Autodesk Inventor part; units mm, degrees
ref_plane "YZ Plane" through (0, 0, 0) normal (1, 0, 0) x (0, 1, 0)
ref_plane "XZ Plane" through (0, 0, 0) normal (0, 1, 0) x (-1, 0, 0)
ref_plane "XY Plane" through (0, 0, 0) normal (0, 0, 1) x (1, 0, 0)
sketch "Sketch1" plane through (0, 0, 0) normal (0, 0, 1) x (1, 0, 0)
  arc A0 (-1.508, 2.794) -> (-1.508, -2.794) centre (0, 0) ccw
  line L0 (-3.175, 0) -> (0, 0) construction
  line L1 (0, 0) -> (3.175, 0) construction
  line L2 (-1.508, 2.794) -> (1.508, 2.794)
  line L3 (-1.508, -2.794) -> (1.508, -2.794)
  arc A1 (1.508, 2.794) -> (-1.508, 2.794) centre (0, 0) ccw construction
  arc A2 (1.508, -2.794) -> (1.508, 2.794) centre (0, 0) ccw
  arc A3 (-1.508, -2.794) -> (1.508, -2.794) centre (0, 0) ccw construction
  circle A4 centre (0, 0) radius 3.429 construction
  circle A5 centre (0, 0) radius 4.064
  circle A6 centre (0, 0) radius 11.1125
  dimension "d1" = 2.794
  dimension "d2" = 3.175
  dimension "d3" = 6.858
  dimension "d5" = 0.635
  dimension "d6" = 22.225
extrude "Extrusion1" add sketch "Sketch1" along normal blind 3.048 contours A5 | A6
sketch "Sketch2" plane through (0, 0, 3.048) normal (0, 0, 1) x (1, 0, 0)
  circle A0 centre (0, 0) radius 11.1125
  arc A1 (-1.508, 2.794) -> (-1.508, -2.794) centre (0, 0) ccw
extrude "Extrusion2" add sketch "Sketch2" along normal blind 3.175
hole "Hole1" at (0, 0, 3.048) direction (0, 0, 1) diameter 3.302 depth 25.4 tip angle 118
sketch "Sketch3" plane through (0, 0, 6.223) normal (0, 0, 1) x (1, 0, 0)
  circle A0 centre (0, 0) radius 11.1125
  circle A1 centre (0, 0) radius 3.429
  circle A2 centre (0, 0) radius 4.064
  dimension "d18" = 6.858
  dimension "d19" = 0.635
extrude "Extrusion3" add sketch "Sketch3" along normal blind 6.1341 contours A0
chamfer "Chamfer1" distance 6.35 distance2 12.3571 1 edges at (-11.1125, 0, 0) measured on face at (0.4465, -5.5398, 0)
sketch "Sketch6" plane through (0, 0, 12.3571) normal (0, 0, 1) x (1, 0, 0)
  circle A0 centre (0, 0) radius 11.1125
  circle A1 centre (0, 0) radius 6.35
  circle A2 centre (0, 0) radius 8.7312
  dimension "d38" = 12.7
  dimension "d52" = 2.3813
  dimension "d53" = 2.3813
extrude "Extrusion5" add sketch "Sketch6" along normal blind 4.9784 contours A2
sketch "Sketch7" plane through (0, 0, 0) normal (1, 0, 0) x (0, 1, 0)
  line L0 (-6.35, 17.3355) -> (6.35, 17.3355)
  line L1 (6.35, 12.3571) -> (-6.35, 12.3571)
  line L2 (0, 0) -> (0, 12.3571) construction
  line L3 (0, 12.3571) -> (0, 17.3355) construction
  point P0 (0, 14.8463)
hole "Hole3" at (0, 0, 14.8463) direction (-1, 0, 0) diameter 2.159 end through all
sketch "Sketch8" plane through (0, 0, 12.3571) normal (0, 0, 1) x (1, 0, 0)
  circle A0 centre (0, 0) radius 11.1125
  circle A1 centre (0, 0) radius 8.7312
  line L0 (-10.3187, 4.1244) -> (-10.3188, -4.1244)
  line L1 (-11.1125, 0) -> (0, 0)
  dimension "d49" = 0.7937
extrude "Extrusion6" cut sketch "Sketch8" against normal through all contours L0 L1 A0 | A0 L1 L0
mirror "Mirror2" about plane through (0, 0, 0) normal (1, 0, 0) of "Hole3", "Extrusion6"
ref_plane "Work Plane2" through (0, 0, 4.953) normal (0, 0, -1) x (-1, 0, 0)
sketch "Sketch9" plane through (0, 0, 4.953) normal (0, 0, -1) x (-1, 0, 0)
  point P0 (0, 0)
equation "\"d52\" = d53"
properties part number "Pneumatic Connector -Actuator Side"
Verification items for the finished model (mm, model axes). A direction names the side the tool comes from. Give positions to 0.01 mm unless a question says otherwise; leave off trailing zeros. Loops run counter-clockwise (first coordinate to the right, second up) from the corner with the lowest first, then second, coordinate; pieces in that order, holes last.
1) Depth check by flat-ended pin: pin 1 Ø1.5 at (y, z) = (-7.5, 8) entering from -X; pin 2 Ø1.9 at (y, z) = (0, 14.85) entering from +X; pin 3 Ø6.5 at (x, y) = (-0.5, -1.5) entering from +Z; pin 4 Ø2.5 at (y, z) = (0, 14.85) entering from -X. Enter the tip coordinate at first touch or a pass-through.
2) Sectioned sample at D-D, the plane z = 4.5. Enter the section's corners in (x, y).
3) Sectioned sample at A-A, the plane y = 0. Count the separate pieces of the cut face and the enclosed holes in it, then the cut area to 3 significant figures.
4) Sectioned sample at C-C, the plane z = 14.5. Enter the section's corners in (x, y), then the cut area to 3 significant figures.
5) Draft check along Y on faces 1 (the flat face through (-6, -3, 17.336)), 2 (the cylindrical face through (7.512, -0.413, 13.849)), 3 (the cylindrical face through (0.632, 1.525, 4.658)), 4 (the conical face through (6.07, -2.52, 3.52)). Enter one of: pulls with the +Y half, pulls with the -Y half, needs draft (parallel to the pull), parting line crosses it, or undercut.
6) Set-up check for faces 5 (the cylindrical face through (-3.175, -0.048, 1.503)), 6 (the flat face through (-7, 6, 12.357)), 7 (the flat face through (0, -3, 0)): record each of +Z, -Z, +X, -X, +Y, -Y from which the full face is reachable in a straight line by a thin tool's end or side.
7) Thickness scan on line 1 along Y through (x, z) = (0, 14.95); line 2 along X through (y, z) = (1.25, 8); line 3 along Y through (x, z) = (-2, 3). Record the ranges inside material, lowest first.
Answers:
1. pin 1: stops at x = -5.94
1. pin 2: passes through
1. pin 3: stops at z = 12.36
1. pin 4: stops at x = -8.73
2. outline: circle Ø14.15 at (0, 0); hole circle Ø3.3 at (0, 0)
3. separate pieces: 4
3. enclosed holes: 0
3. area: 129 mm2
4. outline: (-8.67, -1.02) arc R8.73 ccw to (8.67, -1.02) - (6.27, -1.02) arc R6.35 cw to (-6.27, -1.02) - close; (-8.67, 1.02) - (-6.27, 1.02) arc R6.35 cw to (6.27, 1.02) - (8.67, 1.02) arc R8.73 ccw to start
4. area: 103 mm2
5. face 1: needs draft
5. face 2: undercut
5. face 3: undercut
5. face 4: parting line crosses it
6. face 5: -Z
6. face 6: +Z
6. face 7: -Z, +X, -X, +Y, -Y
7. line 1: y = -8.73 to -6.35, 6.35 to 8.73
7. line 2: x = -8.79 to -3.87, 3.87 to 8.79
7. line 3: y = -5.98 to -2.47, 2.47 to 5.98
